The model under review builds one solid part; all positions refer to its coordinate system, in mm. A direction names the side the tool comes from. Round coordinates to 2 decimals unless told otherwise and drop trailing zeros. Write each loop counter-clockwise with the first axis right and the second up, starting at its lowest first coordinate (ties: lowest second). Pieces come first, ordered by that corner, then holes.
Item 1: Add section A-A (y = 6). Give the boundary of the cut face in (x, z), plus the area to 3 significant figures.
Item 2: Machinability: for faces 5 (the face through (-1.42, 5.916, 2.414)), 6 (the face through (-1.3, 12, 1.4)), which of the approach directions +Z, -Z, +X, -X, +Y, -Y give a long, thin tool a straight path to every point of the face, cutting with its end or side? Answer none if there is none.
Item 3: To check wall thickness, follow L1, parallel to Y at x = -0.5, z = 2.75; L2, parallel to Z at x = -1.05, y = 6.25; L3, parallel to Z at x = -0.65, y = 7.75. State the ranges of each line that lie inside material, in increasing order.
Item 4: Add section B-B (z = 0). Give the boundary of the cut face in (x, y).
Item 5: Add section D-D (z = -2). Give the boundary of the cut face in (x, y).
Item 6: Add section C-C (x = -1.85). Give the boundary of the cut face in (y, z), plus the area to 3 significant figures.
Item 7: Draft analysis for pull direction Z (two halves, no side actions). For faces 1 (the face through (-1.5, 4.93, 0.07)), 2 (the face through (-2.8, 6, 0)), 3 (the face through (0, 10, 0)), 4 (the face through (-1.38, 5.916, -2.436)), state which applies: +Z half, -Z half, draft (parallel to the pull), parting line (faces both ways), or undercut.
Item 8: Clearance check with flat-ended pins moving along their axes: pin 1 Ø0.9 at (x, z) = (-0.5, 0.5) entering from -Y; pin 2 Ø2 at (x, y) = (-2, 8.5) entering from +Z. State where each tip first meets the part, or that it passes through.
```python
from build123d import *

# Parameters (mm, degrees)
BOSS_EXTRUDE1_DEPTH = 12
SKETCH2_R           = 1.5
BOSS_EXTRUDE2_DEPTH = 5.9
SKETCH3_R           = 1.5
CUT_EXTRUDE1_DEPTH  = 10
CHAMFER1_SIZE       = 0.5


with BuildPart() as part:
    # Sketch1 → Boss-Extrude1 (new body)
    with BuildSketch(Plane(origin=(0, 0, 0), x_dir=(1, 0, 0), z_dir=(0, 1, 0))):
        Polygon((0, -3.233161507), (2.8, -1.616580754), (2.8, 1.616580754), (0, 3.233161507), (-2.8, 1.616580754), (-2.8, -1.616580754), align=None)
    extrude(amount=BOSS_EXTRUDE1_DEPTH)

    # Sketch2 → Boss-Extrude2 (add)
    with BuildSketch(Plane(origin=(0, 12, 0), x_dir=(1, 0, 0), z_dir=(0, 1, 0))):
        Circle(SKETCH2_R)
    extrude(amount=BOSS_EXTRUDE2_DEPTH)

    # Sketch3 → Cut-Extrude1 (cut)
    with BuildSketch(Plane.XZ):
        Circle(SKETCH3_R)
    extrude(amount=-CUT_EXTRUDE1_DEPTH, mode=Mode.SUBTRACT)

    # Chamfer1
    chamfer1_edges = [part.edges().sort_by_distance(p)[0] for p in [
        (-1.5, 17.9, 0),
    ]]
    chamfer(chamfer1_edges, length=CHAMFER1_SIZE)


solid = part.part
```
Numbers:
1. outline: (-2.8, -1.62) - (0, -3.23) - (2.8, -1.62) - (2.8, 1.62) - (0, 3.23) - (-2.8, 1.62) - close; hole circle Ø3 at (0, 0)
1. area: 20.1 mm2
2. face 5: +Z, -X, +Y, -Y
2. face 6: +Y
3. L1: y = 0 to 12
3. L2: z = -2.63 to -1.07, 1.07 to 2.63
3. L3: z = -2.86 to -1.35, 1.35 to 2.86
4. outline: (-2.8, 0) - (-1.5, 0) - (-1.5, 10) - (1.5, 10) - (1.5, 0) - (2.8, 0) - (2.8, 12) - (1.5, 12) - (1.5, 17.4) - (1, 17.9) - (-1, 17.9) - (-1.5, 17.4) - (-1.5, 12) - (-2.8, 12) - close
5. outline: (-2.14, 0) - (2.14, 0) - (2.14, 12) - (-2.14, 12) - close
6. outline: (0, -2.17) - (12, -2.17) - (12, 2.17) - (0, 2.17) - close
6. area: 52.0 mm2
7. face 1: undercut
7. face 2: draft
7. face 3: undercut
7. face 4: -Z half
8. pin 1: stops at y = 10
8. pin 2: stops at z = 2.66
